Source: CAD feature listing. Evaluate the final solid. Frame: model axes, mm. A direction names the side the tool comes from. Coordinates: 2 decimals unless noted, no trailing zeros. Loops run counter-clockwise (first coordinate to the right, second up) from the corner with the lowest first, then second, coordinate; pieces in that order, holes last.
Item 1: Pull-direction query (Y, two-part tool) for faces 1 (the conical face through (32.2, 15.6, -3.5)), 2 (the flat face through (60, 0, 0)), 3 (the cylindrical face through (29.423, -6.675, 3.755)); classes: +Y half, -Y half, draft (parallel to the pull), parting line (faces both ways), or undercut.
Item 2: Section query C-C, the plane x = 56. Return the cut outline in (y, z).
Item 3: Pin query (flat end, axial travel): pin 1 Ø5 at (y, z) = (-1, -6.5) entering from -X; pin 2 Ø10 at (x, y) = (33.5, 7) entering from +Z; pin 3 Ø1 at (x, y) = (38.5, -1) entering from +Z; pin 4 Ø6 at (x, y) = (41.5, -8.5) entering from -Z. Return the tip coordinate at first contact, or that it passes through.
Item 4: Reachability of faces 4 (the cylindrical face through (31.356, -15.768, -5.745)), 5 (the cylindrical face through (58.381, -0.66, -14.985)), 6 (the cylindrical face through (70.226, 10.648, -13.887)) from +Z, -Z, +X, -X, +Y, -Y: full face, straight path, thin tool, end or side. Return the list, or none.
Item 5: Line query: probe 1 along Y at (x, z) = (63.5, 0); probe 2 along Z at (x, y) = (17.5, -14); probe 3 along Z at (x, y) = (69.75, 0). Output: solid intervals per line, ascending.
Item 6: Section query B-B, the plane x = 17.5. Return the cut outline in (y, z), then the cut area to 3 significant figures.
```python
from build123d import *

# Parameters (mm, degrees)
F2_R     = 15
F3_DEPTH = 19
F4_R     = 12.5
F5_DEPTH = 25
F6_R     = 1.5


with BuildPart() as f1:
    # F0 (on Front) → F1 (revolve)
    with BuildSketch(Plane.XZ):
        Polygon((0, 17.5), (0, 0), (60, 0), (60, 10), (75, 10), (75, 15), (72, 15), (72, 17.5), (67, 17.5), (67, 15), (50, 15), (5, 17.5), align=None)
    revolve(axis=Axis((30, 0, 0), (1, 0, 0)))

    # F2 (on Front) → F3 (join)
    with BuildSketch(Plane.XZ):
        with Locations((17.5, 0)):
            Circle(F2_R)
    extrude(amount=F3_DEPTH)

    # F4 (on face) → F5 (cut)
    with BuildSketch(Plane.XZ.offset(19)):
        with Locations((17.5, 0)):
            Circle(F4_R)
    extrude(amount=-F5_DEPTH, mode=Mode.SUBTRACT)

    # F6
    f6_edges = [f1.edges().sort_by_distance(p)[0] for p in [
        (2.5, -19, 0),
        (0, 0, -17.5),
        (67, 0, -17.5),
        (75, 0, -10),
        (72, 0, -15),
    ]]
    fillet(f6_edges, radius=F6_R)


solid = f1.part
```
Verdict:
1. face 1: parting line
1. face 2: undercut
1. face 3: draft
2. outline: circle Ø30 at (0, 0)
3. pin 1: stops at x = 0
3. pin 2: stops at z = 15.85
3. pin 3: stops at z = 15.65
3. pin 4: stops at z = -14.48
4. face 4: -Y
4. face 5: none
4. face 6: +X
5. probe 1: y = -15 to -10, 10 to 15
5. probe 2: z = -15 to -12.5, 12.5 to 15
5. probe 3: z = -17.5 to -10, 10 to 17.5
6. outline: (-19, -13.5) arc R1.5 ccw to (-17.5, -15) - (-7.58, -15) arc R16.81 ccw (long way) to (-7.58, 15) - (-17.5, 15) arc R1.5 ccw to (-19, 13.5) - (-19, 12.5) - (6, 12.5) - (6, -12.5) - (-19, -12.5) - close
6. area: 406 mm2
